Design review of the part built by this model. Coordinates are the model's own, in mm. A direction names the side the tool comes from. Coordinates: 2 decimals unless noted, no trailing zeros. Order: outer loops, then holes, each group sorted by start corner. A loop starts at its lowest first (then second) coordinate and runs counter-clockwise, first axis right, second up.
from build123d import *

# Parameters (mm, degrees)
F0_W     = 116
F0_H     = 84
F1_DEPTH = 10
F2_SIZE  = 5
F3_T     = -2.5


with BuildPart() as f1:
    # F0 (on Top) → F1 (new body)
    with BuildSketch(Plane.XY):
        with Locations((-2.746954, 0.195384)):
            Rectangle(F0_W, F0_H)
    extrude(amount=-F1_DEPTH)

    # F2
    f2_edges = [f1.edges().sort_by_distance(p)[0] for p in [
        (55.253046, -41.804616, -5),
        (-60.746954, -41.804616, -5),
        (55.253046, 42.195384, -5),
        (-60.746954, 42.195384, -5),
    ]]
    chamfer(f2_edges, length=F2_SIZE)

    # F3
    f3_openings = [f1.faces().sort_by_distance(p)[0] for p in [
        (-2.746954, 0.195384, 0),
    ]]
    offset(amount=F3_T, openings=f3_openings)


solid = f1.part
1. Add section A-A (x = 14). Give the boundary of the cut face in (y, z), and give its area (4 significant figures).
2. Insertion check: pin 1 (2 mm diameter, centred on x = -26, y = 25.5, fed in from +Z). The pin has a flat end and moves straight along its axis. Give the tip position at first contact, or say it passes through.
3. Add section C-C (y = 1). Give the boundary of the cut face in (x, z).
4. Add section B-B (z = -5.5). Give the boundary of the cut face in (x, y), and give its area (3 significant figures).
5. For faces 5 (the flat face through (-58.21, -39.34, -4.93)), 6 (the flat face through (-56.454, -37.562, -3.698)), list the 3-axis set-ups (+Z, -Z, +X, -X, +Y, -Y) from which the entire face can be reached by the end or side of a thin tool; tool diameter is ignored.
6. Mouldability with a two-part tool opening along Y and no side actions: class faces 1 (the flat face through (-3, 39.695, -4)), 2 (the flat face through (-3, -41.805, -5)), 3 (the flat face through (51.01, -37.51, -3.7)), 4 (the flat face through (-60.747, 0, -5)) as pulls with the +Y half, pulls with the -Y half, needs draft (parallel to the pull), parting line crosses it, or undercut.
7. To check wall thickness, follow line 1 (Y direction, x = -24, z = -5.5); line 2 (X direction, y = -3.5, z = -2.25); line 3 (Z direction, x = -29, y = 7). State the ranges of each line that lie inside material, in increasing order.
Solution:
1. outline: (-41.8, -10) - (42.2, -10) - (42.2, 0) - (39.7, 0) - (39.7, -7.5) - (-39.3, -7.5) - (-39.3, 0) - (-41.8, 0) - close
1. area: 247.5 mm2
2. pin 1: stops at z = -7.5
3. outline: (-60.75, -10) - (55.25, -10) - (55.25, 0) - (52.75, 0) - (52.75, -7.5) - (-58.25, -7.5) - (-58.25, 0) - (-60.75, 0) - close
4. outline: (-60.75, -36.8) - (-55.75, -41.8) - (50.25, -41.8) - (55.25, -36.8) - (55.25, 37.2) - (50.25, 42.2) - (-55.75, 42.2) - (-60.75, 37.2) - close; hole (-58.25, -35.77) - (-54.71, -39.3) - (49.22, -39.3) - (52.75, -35.77) - (52.75, 36.16) - (49.22, 39.7) - (-54.71, 39.7) - (-58.25, 36.16) - close
4. area: 950 mm2
5. face 5: +Z, -Z, -X, -Y
5. face 6: +Z
6. face 1: undercut
6. face 2: pulls with the -Y half
6. face 3: undercut
6. face 4: needs draft
7. line 1: y = -41.8 to -39.3, 39.7 to 42.2
7. line 2: x = -60.75 to -58.25, 52.75 to 55.25
7. line 3: z = -10 to -7.5
